Could you check a few things on this model? Use its own coordinates, in mm. A direction names the side the tool comes from. Give positions to 0.01 mm unless a question says otherwise; leave off trailing zeros. Order: outer loops, then holes, each group sorted by start corner. A loop starts at its lowest first (then second) coordinate and runs counter-clockwise, first axis right, second up. Notation, with made-up numbers: (65.5, -6.75) -> (100.5, -6.75) arc R11 cw to (100.5, 8.25) -> close; hole circle Ø10 at (5.5, 13). An arc over 180 degrees is marked (long way). Answer as CSV lines item,"result". Start each with the question number.
(1) Will these pins go through, and if not, where does the flat tip stop? pin 1 Ø3 at (x, z) = (45, -13) entering from +Y; pin 2 Ø3 at (y, z) = (6, -68.5) entering from -X.
(2) I want a section at B-B (y = 5.75). Give the number of separate pieces and of enclosed holes in the cut face, plus the area to 3 significant figures.
(3) I want a section at A-A (z = -175). Please give me the cut outline in (x, y), plus the area to 3 significant figures.
(4) I need wall thicknesses on L1, parallel to X at y = 3.75, z = -13; L2, parallel to X at y = 6.5, z = 13; L3, parallel to X at y = 0.5, z = -354.5. Which ranges of each line are inside material? Lowest first, please.
(5) On a 3-axis mill with a long thin cutter (end or side, diameter ignored), from which of +Z, -Z, +X, -X, +Y, -Y can I reach the whole of each face in a straight line? I mean faces 1 (the face through (1, 0, -207)), 2 (the face through (43, 5, -20)), 3 (the face through (-34.835, 5, -227)). Say none if no direction works.
Autodesk Inventor part; units mm, degrees
ref_plane "YZ Plane" through (0, 0, 0) normal (1, 0, 0) x (0, 1, 0)
ref_plane "XZ Plane" through (0, 0, 0) normal (0, 1, 0) x (-1, 0, 0)
ref_plane "XY Plane" through (0, 0, 0) normal (0, 0, 1) x (1, 0, 0)
sketch "Szkic3" plane through (0, 0, 0) normal (0, 1, 0) x (-1, 0, 0)
  line L0 (50, 20) -> (-50, 20)
  line L1 (-50, 20) -> (-50, -20)
  line L2 (-50, -20) -> (50, -20)
  line L3 (50, -20) -> (50, 20)
  point P0 (0, 0)
  dimension "d4" = 100
  dimension "d5" = 40
extrude "Wyciągnięcie proste1" add sketch "Szkic3" along normal blind 10
sketch "Szkic4" plane through (0, 10, 0) normal (0, 1, 0) x (1, 0, 0)
  line L0 (50, 20) -> (-50, 20)
  line L1 (35.1646, 20) -> (-34.8354, 20)
  line L2 (-34.8354, 20) -> (-34.8354, 440)
  line L3 (-34.8354, 440) -> (35.1646, 440)
  line L4 (35.1646, 440) -> (35.1646, 20)
  point P0 (0, 0)
  dimension "d8" = 70
  dimension "d9" = 420
extrude "Wyciągnięcie proste2" add sketch "Szkic4" against normal blind 10
sketch "Szkic5" plane through (0, 10, 0) normal (0, 1, 0) x (1, 0, 0)
  line L0 (0, 13) -> (0, -13) construction
  circle A0 centre (-45, 13) radius 2.5
  circle A1 centre (-45, -13) radius 2.5
  circle A2 centre (45, 13) radius 2.5
  circle A3 centre (44.4361, -13) radius 2.5
  line L1 (-45, 13) -> (-11, 13) construction
  line L2 (45, 13) -> (11, 13) construction
  circle A4 centre (-11, 13) radius 2.5
  circle A5 centre (-11, -13) radius 2.5
  circle A6 centre (11, -13) radius 2.5
  circle A7 centre (11, 13) radius 2.5
  point P0 (0, 0)
  dimension "d12" = 26
  dimension "d13" = 5
  dimension "d14" = 5
  dimension "d15" = 5
  dimension "d16" = 5
  dimension "d17" = 34
  dimension "d18" = 34
  dimension "d19" = 5
  dimension "d20" = 5
  dimension "d21" = 5
  dimension "d22" = 5
hole "Otwór1" at (-45, 10, -13) at (-45, 10, 13) at (-11, 10, 13) at (-11, 10, -13) at (11, 10, -13) at (11, 10, 13) at (44.4361, 10, 13) at (45, 10, -13) direction (0, -1, 0) diameter 4.9784 depth 10 tip angle 118
sketch "Szkic6" plane through (0, 10, 0) normal (0, 1, 0) x (1, 0, 0)
  line L0 (35.1646, 440) -> (35.1646, 20)
  line L1 (35.1646, 61.6763) -> (-34.8354, 61.6763) construction
  line L2 (-34.8354, 20) -> (-34.8354, 440)
  line L3 (24.5428, 61.6763) -> (-23.3042, 61.6763) construction
  circle A0 centre (-23.3042, 61.6763) radius 4
  circle A1 centre (24.5428, 61.6763) radius 4
  circle A2 centre (-23.3042, 121.6763) radius 4
  circle A3 centre (24.5428, 121.6763) radius 4
  circle A4 centre (-23.3042, 181.6763) radius 4
  circle A5 centre (24.5428, 181.6763) radius 4
  circle A6 centre (-23.3042, 241.6763) radius 4
  circle A7 centre (24.5428, 241.6763) radius 4
  circle A8 centre (-23.3042, 301.6763) radius 4
  circle A9 centre (24.5428, 301.6763) radius 4
  circle A10 centre (-23.3042, 361.6763) radius 4
  circle A11 centre (24.5428, 361.6763) radius 4
  circle A12 centre (-23.3042, 421.6763) radius 4
  circle A13 centre (24.5428, 421.6763) radius 4
  circle A14 centre (0, 61.6763) radius 4
  circle A15 centre (0, 121.6763) radius 4
  circle A16 centre (0, 181.6763) radius 4
  circle A17 centre (0, 241.6763) radius 4
  circle A18 centre (0, 301.6763) radius 4
  circle A19 centre (0, 361.6763) radius 4
  circle A20 centre (0, 421.6763) radius 4
  point P0 (0, 0)
  point P1 (-27.7985, 121.5078)
  point P2 (8.1646, 122)
  point P3 (-27.8354, 182)
  point P4 (8.1646, 182)
  point P5 (-27.8354, 242)
  point P6 (8.1646, 242)
  point P7 (-27.8354, 302)
  point P8 (8.1646, 302)
  point P9 (-27.8354, 362)
  point P10 (8.1646, 362)
  point P11 (-27.8354, 422)
  point P12 (8.1646, 422)
  dimension "d30" = 47.847
  dimension "d45" = 8
  dimension "d49" = 60
  dimension "d61" = 8
  dimension "d64" = 60
  dimension "d76" = 8
  dimension "d79" = 60
hole "Otwór5" at (-23.3042, 10, -61.6763) at (0, 10, -61.6763) at (24.5428, 10, -61.6763) at (-23.3042, 10, -121.6763) at (0, 10, -121.6763) at (24.5428, 10, -121.6763) at (-23.3042, 10, -181.6763) at (0, 10, -181.6763) at (24.5428, 10, -181.6763) at (-23.3042, 10, -241.6763) at (0, 10, -241.6763) at (24.5428, 10, -241.6763) at (-23.3042, 10, -301.6763) at (0, 10, -301.6763) at (24.5428, 10, -301.6763) at (-23.3042, 10, -361.6763) at (0, 10, -361.6763) at (24.5428, 10, -361.6763) at (-23.3042, 10, -421.6763) at (0, 10, -421.6763) at (24.5428, 10, -421.6763) direction (0, -1, 0) diameter 4.9784 depth 50 tip angle 118
properties part number "plaskownik_uchwyt_silownika_L460_W100_H10"
Final values:
1,pin 1,"through"
1,pin 2,"x = -34.84"
2,separate pieces,"1"
2,enclosed holes,"29"
2,area,"32,800 mm²"
3,outline,"(-34.84, 0) -> (35.16, 0) -> (35.16, 10) -> (-34.84, 10) -> close"
3,area,"700 mm²"
4,L1,"-50 to -47.49, -42.51 to -13.49, -8.51 to 8.51, 13.49 to 42.51, 47.49 to 50"
4,L2,"-50 to -47.49, -42.51 to -13.49, -8.51 to 8.51, 13.49 to 41.95, 46.93 to 50"
4,L3,"-34.84 to 35.16"
5,face 1,"+Z, -Z, +X, -X, -Y"
5,face 2,"-Z, +X, +Y, -Y"
5,face 3,"-Z, -X, +Y, -Y"
